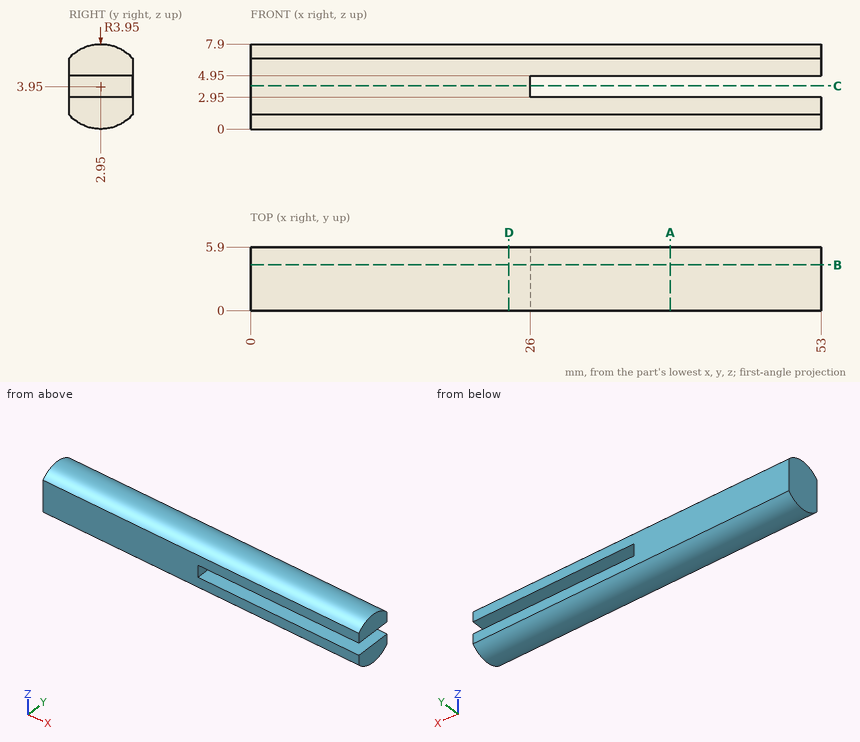
Design review of the part shown in the three views and the two pictorial views. Dimensions are in mm from the part's minimum x, y and z. Round coordinates to 2 decimals unless told otherwise and drop trailing zeros. Write each loop counter-clockwise with the first axis right and the second up, starting at its lowest first coordinate (ties: lowest second). Pieces come first, ordered by that corner, then holes. Notation, with made-up numbers: M 58,30 L 64,30 A21 cw 64,49 Z; hole C 33,53 d4. An arc over 180 degrees is marked long. One line per item, written item: value. Start each with the question number.
1. Take a section at D-D on x = 24. State the section outline as (y, z) points.
2. Take a section at C-C on z = 4. State the section outline as (x, y) points.
3. Take a section at A-A on x = 39. State the section outline as (y, z) points.
4. Clearance check with a flat-ended pin moving along its axis: P1, Ø1, axis at x = 10.5, y = 4, coming from the -Z side. State where the tip first meets the part, or that it passes through.
5. Take a section at B-B on y = 4.25. State the section outline as (x, z) points, then the cut area to 3 significant figures.
6. To check wall thickness, follow probe 1 along X at (y, z) = (3.2, 3); probe 2 along Z at (x, y) = (37, 1.1); probe 3 along Z at (x, y) = (35.5, 0.75). State the ranges of each line that lie inside material, in increasing order. Write a range as from..to.
Computed:
1. outline: M 0,1.32 A3.95 ccw 5.9,1.32 L 5.9,6.58 A3.95 ccw 0,6.58 Z
2. outline: M 0,0 L 26,0 L 26,5.9 L 0,5.9 Z
3. outline: M 0,1.32 A3.95 ccw 5.9,1.32 L 5.9,2.95 L 0,2.95 Z; M 0,4.95 L 5.9,4.95 L 5.9,6.58 A3.95 ccw 0,6.58 Z
4. P1: stops at z = 0.04
5. outline: M 0,0.22 L 53,0.22 L 53,2.95 L 26,2.95 L 26,4.95 L 53,4.95 L 53,7.68 L 0,7.68 Z
5. area: 341 mm²
6. probe 1: x = 0..26
6. probe 2: z = 0.46..2.95, 4.95..7.44
6. probe 3: z = 0.67..2.95, 4.95..7.23
